Source: CAD feature listing. Evaluate the final solid. Frame: model axes, mm. A direction names the side the tool comes from. Give positions to 0.01 mm unless a question says otherwise; leave off trailing zeros. Order: outer loops, then holes, each group sorted by start corner. A loop starts at its lowest first (then second) coordinate and runs counter-clockwise, first axis right, second up.
from build123d import *

# Parameters (mm, degrees)
SKETCH2_W           = 38.1
SKETCH2_H           = 38.1
BOSS_EXTRUDE1_DEPTH = 5.08
BOSS_EXTRUDE3_DEPTH = 38.1
SKETCH5_R           = 12.2084592
CUT_EXTRUDE1_DEPTH  = 39.1
BOSS_EXTRUDE4_DEPTH = 5.08


with BuildPart() as part:
    # Sketch2 → Boss-Extrude1 (new body)
    with BuildSketch(Plane(origin=(0, 0, 0), x_dir=(1, 0, 0), z_dir=(0, 1, 0))):
        Rectangle(SKETCH2_W, SKETCH2_H)
    extrude(amount=BOSS_EXTRUDE1_DEPTH)

    # Sketch3 → Boss-Extrude3 (add, through all)
    with BuildSketch(Plane(origin=(19.05, 0, 0), x_dir=(0, 0, -1), z_dir=(1, 0, 0))):
        with BuildLine():
            Line((-19.05, 5.08), (-14.639336287, 30.094116927))
            ThreePointArc((-14.639336287, 30.094116927), (0, 35.484404044), (14.639336287, 30.094116927))
            Line((14.639336287, 30.094116927), (19.05, 5.08))
            Line((19.05, 5.08), (-19.05, 5.08))
        make_face()
    extrude(amount=-BOSS_EXTRUDE3_DEPTH)

    # Sketch5 → Cut-Extrude1 (cut, through all)
    with BuildSketch(Plane(origin=(19.05, 0, 0), x_dir=(0, 0, -1), z_dir=(1, 0, 0))):
        with Locations((0, 19.05)):
            Circle(SKETCH5_R)
    extrude(amount=-CUT_EXTRUDE1_DEPTH, mode=Mode.SUBTRACT)

    # Sketch6 → Boss-Extrude4 (add)
    with BuildSketch(Plane(origin=(0, 0, -19.05), x_dir=(-1, 0, 0), z_dir=(0, 0, -1))):
        Polygon((19.05, 0), (19.05, -19.05), (0, 0), align=None)
    extrude(amount=-BOSS_EXTRUDE4_DEPTH)


solid = part.part
(1) Draft query along Z for faces 1 (the flat face through (0.267, 17.762, -16.814)), 2 (the cylindrical face through (0.267, 35.483, 0.223)), 3 (the flat face through (-10, -10, -17)), 4 (the cylindrical face through (0.267, 7.132, 2.647)). Return one class per face: +Z half, -Z half, draft (parallel to the pull), parting line (faces both ways), or undercut.
(2) Section B-B, the plane x = -10. Return loops of the section in (y, z), plus the area to 3 significant figures.
(3) Access query for faces 5 (the flat face through (-5, -1, -19.05)), 6 (the flat face through (-12, -7, -13.97)). Directions: +Z, -Z, +X, -X, +Y, -Y. A direction counts if a zero-diameter tool reaches every point of the face in a straight line with its end or side. Return the directions, or none.
(4) Line query: line 1 along Y through (x, z) = (3, 0.5); line 2 along Y through (x, z) = (8, 0); line 3 along Z through (x, y) = (12, 8). Output: solid intervals per line, ascending.
(5) Pin query (flat end, axial travel): pin 1 Ø6 at (x, z) = (-11.5, -7) entering from +Y; pin 2 Ø19 at (x, z) = (-1, 4.5) entering from -Y; pin 3 Ø1.5 at (x, z) = (-3.5, -15) entering from -Y; pin 4 Ø10 at (x, y) = (4, -1) entering from +Z. Return the tip coordinate at first contact, or that it passes through.
(6) Section C-C, the plane y = 28. Return loops of the section in (x, z), plus the area to 3 significant figures.
(7) Section A-A, the plane z = 0. Return loops of the section in (x, y).
(8) Section D-D, the plane x = 4.5. Return loops of the section in (y, z), plus the area to 3 significant figures.
Checks:
1. face 1: -Z half
1. face 2: parting line
1. face 3: draft
1. face 4: undercut
2. outline: (-10, -19.05) - (5.08, -19.05) - (30.09, -14.64) arc R22.57 ccw to (30.09, 14.64) - (5.08, 19.05) - (0, 19.05) - (0, -13.97) - (-10, -13.97) - close; hole circle Ø24.42 at (19.05, 0)
2. area: 727 mm2
3. face 5: -Z, +X, -X, +Y, -Y
3. face 6: +Z, +X, -X, -Y
4. line 1: y = 0 to 6.85, 31.25 to 35.48
4. line 2: y = 0 to 6.84, 31.26 to 35.48
4. line 3: z = -18.54 to -5.19, 5.19 to 18.54
5. pin 1: stops at y = 35.13
5. pin 2: stops at y = 0
5. pin 3: stops at y = -4.25
5. pin 4: stops at z = 19.05
6. outline: (-19.05, -15.01) - (19.05, -15.01) - (19.05, -8.3) - (-19.05, -8.3) - close; (-19.05, 8.3) - (19.05, 8.3) - (19.05, 15.01) - (-19.05, 15.01) - close
6. area: 511 mm2
7. outline: (-19.05, 0) - (19.05, 0) - (19.05, 6.84) - (-19.05, 6.84) - close; (-19.05, 31.26) - (19.05, 31.26) - (19.05, 35.48) - (-19.05, 35.48) - close
8. outline: (0, -19.05) - (5.08, -19.05) - (30.09, -14.64) arc R22.57 ccw to (30.09, 14.64) - (5.08, 19.05) - (0, 19.05) - close; hole circle Ø24.42 at (19.05, 0)
8. area: 676 mm2
